Can you work these out from the model? Positions are in its coordinate system, mm. Face numbers are marked on the shaded views. A direction names the side the tool comes from. Round coordinates to 2 decimals unless told otherwise and drop trailing zeros. Loops run counter-clockwise (first coordinate to the right, second up) from the corner with the lowest first, then second, coordinate; pieces in that order, holes last.
(1) I want a section at D-D on y = 17. Write out the boundary of the cut face in (x, z).
(2) Which directions (+Z, -Z, +X, -X, +Y, -Y) give clear straight access to the entire face, cutting with the end or side of a thin tool? Please do the marked faces 4 and 5.
(3) Thinking about a two-plate mould opening in Y: for the marked faces 1, 2 and 3, which applies, released by +Y, released by -Y, zero draft, split by the parting line, or undercut?
(4) I want a section at C-C on x = -13. Write out the boundary of the cut face in (y, z).
(5) I want a section at A-A on y = 23.5. Write out the boundary of the cut face in (x, z).
(6) If I drill on line 1 along Y through (x, z) = (-25, -8.25); line 2 along Z through (x, y) = (-16, 37); line 3 along Y through (x, z) = (-52.2, 0), over which ranges is the centre line in solid material (lowest first)?
(7) I want a section at B-B on z = -6.5. Write out the boundary of the cut face in (x, y).
(8) Will these pins go through, and if not, where does the flat tip stop? pin 1 Ø8 at (y, z) = (-2, -0.5) entering from +X; pin 2 Ø5 at (y, z) = (17, 6.5) entering from +X; pin 3 Ø12 at (y, z) = (28.5, 6.5) entering from +X.
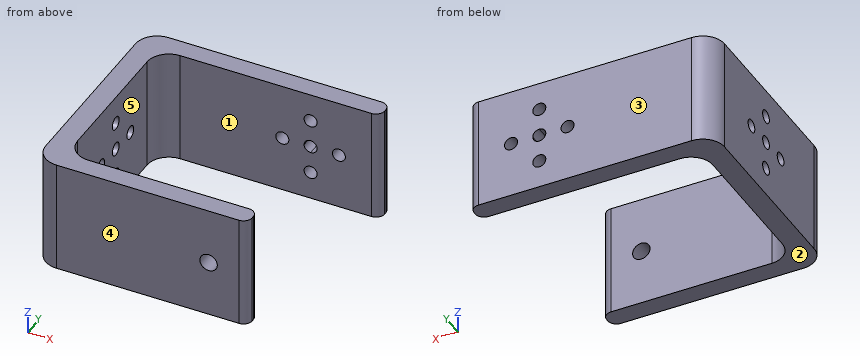
Autodesk Inventor part; units mm, degrees
ref_plane "Work Plane1" through (-47, 34, 13) normal (1, 0, 0) x (0, 0, -1)
ref_plane "Work Plane3" through (-47, -5, 13) normal (0, 1, 0) x (1, 0, 0)
ref_plane "YZ Plane" through (0, 0, 0) normal (1, 0, 0) x (0, 1, 0)
sketch "Sketch1" plane through (0, 0, 0) normal (0, 0, 1) x (1, 0, 0)
  line L0 (0, 0) -> (-51, 0)
  line L1 (-51, 0) -> (-51, 18)
  line L2 (-51, 18) -> (0, 18) construction
  line L3 (-51, 18) -> (-54, 18)
  line L4 (-54, 18) -> (-54, -3)
  line L5 (-54, -3) -> (0, -3)
  line L6 (0, -3) -> (0, 0)
  dimension "d0" = 18
  dimension "d1" = 3
  dimension "d2" = 3
  dimension "d3" = 54
extrude "Extrusion1" add sketch "Sketch1" along normal blind 10
mirror "Mirror1" about plane through (-33.12, 1.38, 0) normal (0, 0, -1) of "Extrusion1"
mirror "Mirror2" about plane through (-51, 18, 0) normal (0, 1, 0) of "Extrusion1", "Mirror1"
sketch "Sketch4" plane through (0, -3, -10) normal (0, 0, -1) x (-1, 0, 0)
  line L0 (0, 3) -> (51, 3)
  line L1 (0, 0) -> (0, 3)
  line L2 (54, 0) -> (0, 0)
  line L3 (54, 42) -> (54, 0)
  line L4 (54, 42) -> (0, 42)
  line L5 (0, 42) -> (0, 39)
  line L6 (0, 39) -> (51, 39)
  line L7 (51, 39) -> (51, 3)
  line L8 (0, 3) -> (51, 3)
  line L9 (0, 0) -> (0, 3)
  line L10 (54, 0) -> (0, 0)
  line L11 (54, 42) -> (54, 0)
  line L12 (54, 42) -> (0, 42)
  line L13 (0, 42) -> (0, 39)
  line L14 (0, 39) -> (51, 39)
  line L15 (51, 39) -> (51, 3)
extrude "Extrusion4" add sketch "Sketch4" along normal blind 5
mirror "Mirror3" about plane through (0, 0, 0) normal (0, 0, 1) of "Extrusion4"
sketch "Sketch11" plane through (-54, -3, -15) normal (0, -1, 0) x (1, 0, 0)
  line L0 (54, 0) -> (54, 30)
  line L1 (54, 30) -> (0, 30)
  line L2 (0, 0) -> (0, 30)
  line L3 (54, 0) -> (0, 0)
  line L4 (54, 0) -> (54, 30)
  line L5 (54, 30) -> (0, 30)
  line L6 (0, 0) -> (0, 30)
  line L7 (54, 0) -> (0, 0)
  point P0 (54, 15)
extrude "Extrusion11" cut sketch "Sketch11" against normal blind 10
sketch "Sketch13" plane through (0, 36, -15) normal (1, 0, 0) x (0, 0, -1)
  line L0 (-30, 3) -> (-28, 3)
  line L1 (-28, 3) -> (-28, -29)
  line L2 (-28, -29) -> (-30, -29)
  line L3 (-30, -29) -> (-30, 3)
  line L4 (-30, -29) -> (0, -29)
  point P0 (-15, -36)
  dimension "d65" = 2
extrude "Extrusion13" cut sketch "Sketch13" against normal up to next
mirror "Mirror4" about plane through (0, 0, 0) normal (0, 0, 1) of "Extrusion13"
sketch "Sketch14" plane through (-54, 7, 13) normal (-1, 0, 0) x (0, 0, 1)
  line L0 (-26, 32) -> (-26, 0)
  line L1 (-26, 0) -> (0, 0)
  line L2 (0, 32) -> (-26, 32)
  circle A0 centre (-13, 10) radius 6.5 construction
  line L3 (-13, 10) -> (-26, 10) construction
  line L4 (-13, 10) -> (-13, 32) construction
  circle A1 centre (-13, 10) radius 1.5
  circle A2 centre (-13, 16.5) radius 1.5
  point P0 (-13, -7)
  point P1 (-13, 0)
  dimension "d68" = 13
  dimension "d69" = 22
  dimension "d71" = 3
  dimension "d72" = 3
extrude "Extrusion14" cut sketch "Sketch14" against normal up to next
pattern_circular "Circular Pattern6" count 4 over 360 about axis through (-54, 17, 0) along (1, 0, 0) of "Extrusion14"
sketch "Sketch15" plane through (-51, 36, 13) normal (0, -1, 0) x (1, 0, 0)
  line L0 (51, -26) -> (51, 0)
  line L1 (51, 0) -> (0, 0)
  circle A0 centre (35, -13) radius 6.5 construction
  line L2 (35, -13) -> (35, 0) construction
  circle A1 centre (35, -6.5) radius 1.5
  circle A2 centre (35, -13) radius 1.5
  point P0 (51, -13)
  point P1 (51, -13)
  dimension "d78" = 13
  dimension "d79" = 16
  dimension "d80" = 3
  dimension "d81" = 3
extrude "Extrusion15" cut sketch "Sketch15" against normal up to next
pattern_circular "Circular Pattern7" count 4 over 360 about axis through (-16, 36, 0) along (0, 1, 0) of "Extrusion15"
sketch "Sketch16" plane through (-54, 7, -15) normal (0, -1, 0) x (1, 0, 0)
  line L0 (0, 2) -> (3, 2)
  line L1 (3, 28) -> (3, 2)
  line L2 (3, 28) -> (0, 28)
  line L3 (0, 2) -> (0, 28)
  line L4 (0, 2) -> (3, 2)
  line L5 (3, 28) -> (3, 2)
  line L6 (3, 28) -> (0, 28)
  line L7 (0, 2) -> (0, 28)
  point P0 (54, 15)
extrude "Extrusion16" add sketch "Sketch16" along normal blind 14
ref_plane "Work Plane1" through (-47, 34, 13) normal (1, 0, 0) x (0, 0, -1)
sketch "Sketch17" plane through (-47, 34, 13) normal (1, 0, 0) x (0, 0, -1)
  line L0 (0, 0) -> (0, -41)
  line L1 (26, -41) -> (0, -41)
  line L2 (0, -41) -> (0, -39)
  line L3 (0, -39) -> (26, -39)
  line L4 (26, -39) -> (26, -41)
  point P0 (13, -34)
  dimension "d92" = 2
extrude "Extrusion17" add sketch "Sketch17" along normal blind 40
ref_plane "Work Plane3" through (-47, -5, 13) normal (0, 1, 0) x (1, 0, 0)
sketch "Sketch18" plane through (-47, -5, 13) normal (0, 1, 0) x (1, 0, 0)
  circle A0 centre (31, 13) radius 1.5
  circle A1 centre (31, 13) radius 2
  point P0 (47, 13)
  dimension "d95" = 4
extrude "Extrusion18" cut sketch "Sketch18" against normal up to next contours A0 | A1
sketch "Sketch23" plane through (0, 36, 13) normal (0, 0, 1) x (1, 0, 0)
  line L0 (0, 0) -> (-51, 0)
  line L1 (-54, 3) -> (0, 3)
  line L2 (-54, -43) -> (-54, 3)
  line L3 (-7, -43) -> (-54, -43)
  line L4 (-47, -41) -> (-7, -41)
  line L5 (-51, 0) -> (-51, -43)
  line L6 (0, 0) -> (-51, 0)
  line L7 (0, 3) -> (0, 0)
  line L8 (-54, 3) -> (0, 3)
  line L9 (-54, -43) -> (-54, 3)
  line L10 (-51, -43) -> (-54, -43)
  line L11 (0, 0) -> (-54, 0)
  line L12 (-54, 0) -> (-54, 4.5)
  line L13 (-54, 4.5) -> (0, 4.5)
  line L14 (0, 4.5) -> (0, 0)
  line L15 (-7, -41) -> (-54, -41)
  line L16 (-54, -41) -> (-54, -45.5)
  line L17 (-54, -45.5) -> (-7, -45.5)
  line L18 (-7, -45.5) -> (-7, -41)
  point P0 (0, -36)
  dimension "d110" = 3
  dimension "d111" = 2
  dimension "d112" = 1.5
  dimension "d113" = 2.5
sketch "Sketch24" plane through (-54, 39, 13) normal (0, 1, 0) x (1, 0, 0)
  circle A0 centre (38, 19.5) radius 1.5
  circle A1 centre (44.5, 13) radius 1.5
  circle A2 centre (31.5, 13) radius 1.5
  circle A3 centre (38, 6.5) radius 1.5
  circle A4 centre (38, 13) radius 1.5
  line L0 (54, 26) -> (0, 26)
  line L1 (0, 0) -> (0, 26)
  line L2 (0, 0) -> (54, 0)
  line L3 (54, 0) -> (54, 26)
  point P0 (54, 13)
  dimension "d114" = 26
extrude "Extrusion22" add sketch "Sketch23" against normal up to surface (26 mm away) contours L0 L11 L2 L1 L7 | L1 L12 L13 L14 | L15 L4 L18 L3 L5 | L5 L3 L2 L15 | L3 L18 L17 L16
sketch "Sketch25" plane through (-51, 36, 13) normal (0, 0, 1) x (1, 0, 0)
  line L0 (-3, 4.5) -> (-3, -45.5)
  line L1 (-3, -45.5) -> (44, -45.5)
  line L2 (44, -41) -> (44, -45.5)
  line L3 (44, -41) -> (0, -41)
  line L4 (0, 0) -> (0, -41)
  line L5 (51, 0) -> (0, 0)
  line L6 (51, 4.5) -> (51, 0)
  line L7 (51, 4.5) -> (-3, 4.5)
  point P0 (51, -36)
  dimension "d117" = 3
sketch "Sketch26" plane through (-54, -9.5, -13) normal (-1, 0, 0) x (0, 0, 1)
  line L0 (0, 0) -> (0, 50)
  line L1 (26, 0) -> (0, 0)
  line L2 (26, 50) -> (26, 0)
  line L3 (26, 50) -> (0, 50)
  circle A0 centre (13, 20) radius 1.5
  circle A1 centre (19.5, 26.5) radius 1.5
  circle A2 centre (6.5, 26.5) radius 1.5
  circle A3 centre (13, 26.5) radius 1.5
  circle A4 centre (13, 33) radius 1.5
  line L4 (0, 0) -> (0, 50)
  line L5 (26, 0) -> (0, 0)
  line L6 (26, 50) -> (26, 0)
  circle A5 centre (13, 20) radius 1.5
  circle A6 centre (19.5, 26.5) radius 1.5
  circle A7 centre (6.5, 26.5) radius 1.5
  circle A8 centre (13, 26.5) radius 1.5
  circle A9 centre (13, 33) radius 1.5
  line L7 (26, 50) -> (0, 50)
  point P0 (13, 9.5)
extrude "Extrusion23" add sketch "Sketch26" along normal blind 2
sketch "Sketch27" plane through (0, 40.5, 13) normal (0, 1, 0) x (1, 0, 0)
  line L0 (-56, 26) -> (0, 26)
  line L1 (0, 0) -> (0, 26)
  circle A0 centre (-16, 13) radius 6.5 construction
  circle A1 centre (-16, 19.5) radius 1.5
  circle A2 centre (-16, 13) radius 1.5
  line L2 (-16, 13) -> (0, 13) construction
  line L3 (-16, 13) -> (-16, 26) construction
  dimension "d121" = 13
  dimension "d120" = 3
  dimension "d122" = 3
  dimension "d123" = 16
extrude "Extrusion24" cut sketch "Sketch27" against normal up to surface (4.5 mm away)
pattern_circular "Circular Pattern8" count 4 over 360 about axis through (-16, 40.5, 0) along (0, -1, 0) of "Extrusion24"
sketch "Sketch28" plane through (-51, -5, 13) normal (0, 1, 0) x (1, 0, 0)
  circle A0 centre (35, 13) radius 1.5
  circle A1 centre (35, 13) radius 2
  point P0 (51, 13)
  dimension "d129" = 4
extrude "Extrusion25" cut sketch "Sketch28" against normal up to next contours A0 | A1
fillet "Fillet9" radius 2 4 edges at (-7, -5, 0) (-7, -9.5, 0) (0, 40.5, 0) (0, 36, 0)
fillet "Fillet10" radius 5 2 edges at (-51, -5, 0) (-51, 36, 0)
fillet "Fillet11" radius 5 2 edges at (-56, -9.5, 0) (-56, 40.5, 0)
sketch "Sketch29" plane through (-2, 40.5, 13) normal (0, 1, 0) x (1, 0, 0)
  circle A0 centre (-14, 6.5) radius 1.5
  circle A1 centre (-7.5, 13) radius 1.5
  circle A2 centre (-20.5, 13) radius 1.5
  circle A3 centre (-14, 19.5) radius 1.5
  circle A4 centre (-14, 13) radius 1.5
  line L0 (-49, 0) -> (-49, 26)
  line L1 (0, 0) -> (-49, 0)
  line L2 (0, 26) -> (0, 0)
  line L3 (-49, 26) -> (0, 26)
  line L4 (-62.85, -6.77) -> (-67.62, -6.77)
  line L5 (-117.21, -13.16) -> (-119.57, -13.16)
  point P0 (2, 13)
  point P1 (-65.235, -6.77)
  point P2 (-118.39, -13.16)
  dimension "d135" = 51.235
  dimension "d136" = 104.39
  dimension "d137" = 53.155
sketch "Sketch30" plane through (-46, 36, 13) normal (0, 0, 1) x (1, 0, 0)
  arc A0 (-5, 4.5) -> (-10, -0.5) centre (-5, -0.5) ccw
  line L0 (-10, -40.5) -> (-10, -0.5)
  arc A1 (-10, -40.5) -> (-5, -45.5) centre (-5, -40.5) ccw
  line L1 (-5, -45.5) -> (37, -45.5)
  arc A2 (37, -45.5) -> (39, -43.5) centre (37, -43.5) ccw
  line L2 (39, -43) -> (39, -43.5)
  arc A3 (39, -43) -> (37, -41) centre (37, -43) ccw
  line L3 (37, -41) -> (0, -41)
  arc A4 (-5, -36) -> (0, -41) centre (0, -36) ccw
  line L4 (-5, -5) -> (-5, -36)
  arc A5 (0, 0) -> (-5, -5) centre (0, -5) ccw
  line L5 (44, 0) -> (0, 0)
  arc A6 (44, 0) -> (46, 2) centre (44, 2) ccw
  line L6 (46, 2.5) -> (46, 2)
  arc A7 (46, 2.5) -> (44, 4.5) centre (44, 2.5) ccw
  line L7 (44, 4.5) -> (-5, 4.5)
  circle A8 centre (-21.235, -24.295) radius 1.5
  circle A9 centre (-74.39, -26.06) radius 1.5
  line L8 (28.82, -7.86) -> (31.18, -7.86)
  point P0 (46, -36)
  point P1 (30, -7.86)
  dimension "d138" = 51.235
  dimension "d139" = 104.39
  dimension "d140" = 53.155
sketch "Sketch31" plane through (-2, 40.5, 13) normal (0, 1, 0) x (1, 0, 0)
  circle A0 centre (-14, 6.5) radius 1.5
  circle A1 centre (-7.5, 13) radius 1.5
  circle A2 centre (-20.5, 13) radius 1.5
  circle A3 centre (-14, 19.5) radius 1.5
  circle A4 centre (-14, 13) radius 1.5
  line L0 (-49, 0) -> (-49, 26)
  line L1 (0, 0) -> (-49, 0)
  line L2 (0, 26) -> (0, 0)
  line L3 (-49, 26) -> (0, 26)
  line L4 (-233.9534, -25.52) -> (-233.9534, -21.02)
  point P0 (2, 13)
  point P1 (-118.39, -13.16)
  point P2 (-118.39, -13.16)
  dimension "d141" = 115.5634
sketch "Sketch32" plane through (-46, 36, 13) normal (0, 0, 1) x (1, 0, 0)
  arc A0 (-5, 4.5) -> (-10, -0.5) centre (-5, -0.5) ccw
  line L0 (-10, -40.5) -> (-10, -0.5)
  arc A1 (-10, -40.5) -> (-5, -45.5) centre (-5, -40.5) ccw
  line L1 (-5, -45.5) -> (37, -45.5)
  arc A2 (37, -45.5) -> (39, -43.5) centre (37, -43.5) ccw
  line L2 (39, -43) -> (39, -43.5)
  arc A3 (39, -43) -> (37, -41) centre (37, -43) ccw
  line L3 (37, -41) -> (0, -41)
  arc A4 (-5, -36) -> (0, -41) centre (0, -36) ccw
  line L4 (-5, -5) -> (-5, -36)
  arc A5 (0, 0) -> (-5, -5) centre (0, -5) ccw
  line L5 (44, 0) -> (0, 0)
  arc A6 (44, 0) -> (46, 2) centre (44, 2) ccw
  line L6 (46, 2.5) -> (46, 2)
  arc A7 (46, 2.5) -> (44, 4.5) centre (44, 2.5) ccw
  line L7 (44, 4.5) -> (-5, 4.5)
  arc A8 (-187.9273, -23.2225) -> (-187.9273, -28.8975) centre (-186.9534, -26.06) ccw
  circle A9 centre (-74.39, -26.06) radius 1.18
  point P0 (46, -36)
  point P1 (-189.9534, -26.06)
  dimension "d142" = 115.563
equation "\"d72\" = d71"
properties part number "C_MARK3"
Filled sheet:
1. outline: (-56, -13) - (-51, -13) - (-51, -8) - (-56, -8) - close; (-56, -5) - (-51, -5) - (-51, -1.5) - (-56, -1.5) - close; (-56, 1.5) - (-51, 1.5) - (-51, 5) - (-56, 5) - close; (-56, 8) - (-51, 8) - (-51, 13) - (-56, 13) - close
2. face 4: +Z, -Z, +X, -X, -Y
2. face 5: +Z, -Z, +X
3. face 1: undercut
3. face 2: zero draft
3. face 3: released by +Y
4. outline: (-9.5, -13) - (-5, -13) - (-5, 13) - (-9.5, 13) - close; (36, -13) - (40.5, -13) - (40.5, 13) - (36, 13) - close
5. outline: (-56, -13) - (-51, -13) - (-51, -1.5) - (-56, -1.5) - close; (-56, 1.5) - (-51, 1.5) - (-51, 13) - (-56, 13) - close
6. line 1: y = -9.5 to -5, 36 to 40.5
6. line 2: z = -13 to -8, -5 to -1.5, 1.5 to 5, 8 to 13
6. line 3: y = -9.35 to 9, 12 to 15.5, 18.5 to 22, 25 to 40.35
7. outline: (-56, -4.5) arc R5 ccw to (-51, -9.5) - (-9, -9.5) arc R2 ccw to (-7, -7.5) - (-7, -7) arc R2 ccw to (-9, -5) - (-46, -5) arc R5 cw to (-51, 0) - (-51, 15.5) - (-56, 15.5) - close; (-56, 18.5) - (-51, 18.5) - (-51, 31) arc R5 cw to (-46, 36) - (-17.5, 36) - (-17.5, 40.5) - (-51, 40.5) arc R5 ccw to (-56, 35.5) - close; (-14.5, 36) - (-2, 36) arc R2 ccw to (0, 38) - (0, 38.5) arc R2 ccw to (-2, 40.5) - (-14.5, 40.5) - close
8. pin 1: stops at x = -7.27
8. pin 2: stops at x = -51
8. pin 3: stops at x = -49.57
